Geometry check sheet. Reference: the model listing, model coordinates, mm. Give positions to 0.01 mm unless a question says otherwise; leave off trailing zeros. Order: outer loops, then holes, each group sorted by start corner. A loop starts at its lowest first (then second) coordinate and runs counter-clockwise, first axis right, second up. Notation, with made-up numbers: M 81,78.25 L 109,78.25 A22 ccw 109,93.25 Z; hole C 16.5,-32 d7. An arc over 180 degrees is marked long. Answer as a JSON object with one key per item and string values. Group by question number.
Autodesk Inventor part; units mm, degrees
ref_plane "YZ Plane" through (0, 0, 0) normal (1, 0, 0) x (0, 1, 0)
ref_plane "XZ Plane" through (0, 0, 0) normal (0, 1, 0) x (-1, 0, 0)
ref_plane "XY Plane" through (0, 0, 0) normal (0, 0, 1) x (1, 0, 0)
sketch "Sketch1" plane through (0, 0, 0) normal (0, 0, 1) x (1, 0, 0)
  line L0 (0, -7) -> (208, -7)
  line L1 (209, -8) -> (209, -30)
  line L2 (208, -31) -> (0, -31)
  line L3 (-1, -30) -> (-1, -8)
  circle A0 centre (38.25, -10.75) radius 1.75
  circle A1 centre (58.75, -10.75) radius 1.75
  circle A2 centre (149.25, -10.75) radius 1.75
  circle A3 centre (169.75, -10.75) radius 1.75
  circle A4 centre (38.25, -40.75) radius 1.75
  circle A5 centre (58.75, -40.75) radius 1.75
  circle A6 centre (149.25, -40.75) radius 1.75
  circle A7 centre (169.75, -40.75) radius 1.75
  arc A8 (0, -7) -> (-1, -8) centre (0, -8) ccw
  arc A9 (-1, -30) -> (0, -31) centre (0, -30) ccw
  arc A10 (208, -31) -> (209, -30) centre (208, -30) ccw
  arc A11 (209, -8) -> (208, -7) centre (208, -8) ccw
  point P0 (0, 0)
  point P1 (209, -31)
  point P2 (209, -7)
  point P3 (-1, -31)
  dimension "d0" = 210
  dimension "d1" = 24
  dimension "d10" = 111
  dimension "d13" = 30
  dimension "d16" = 1
extrude "Extrusion1" add sketch "Sketch1" along normal blind 2 contours L0 A11 L1 A10 L2 A9 L3 A8 | A0 | A1 | A2 | A3
sketch "Sketch2" plane through (0, 0, 2) normal (0, 0, 1) x (1, 0, 0)
  line L0 (209, -30) -> (209, -8)
  line L1 (209, -19) -> (-1, -19) construction
  line L2 (-1, -8) -> (-1, -30)
  line L3 (235.9536, -47.1551) -> (247.5417, -11.4905)
  line L4 (235.9536, -47.1551) -> (273.4536, -47.1551) construction
  line L5 (235.9536, -47.1551) -> (237.8557, -47.7731)
  line L6 (235.9536, -47.1551) -> (237.9536, -47.1551) construction
  line L7 (237.8557, -47.7731) -> (249.4438, -12.1085)
  line L8 (249.4438, -12.1085) -> (247.5417, -11.4905)
  line L9 (249.4438, -12.1085) -> (271.3181, -19.2159)
  line L10 (271.3181, -19.2159) -> (259.73, -54.8805)
  line L11 (259.73, -54.8805) -> (261.6321, -55.4986)
  line L12 (261.6321, -55.4986) -> (273.2202, -19.8339)
  line L13 (273.2202, -19.8339) -> (271.3181, -19.2159)
  line L14 (265.5241, -37.0482) -> (243.6498, -29.9408)
  line L15 (177.3204, -33.4945) -> (331.8534, -33.4945)
  line L16 (244.4446, -27.4945) -> (242.5425, -26.8765)
  line L17 (238.4427, -39.4945) -> (240.3448, -40.1125)
  line L18 (244.4446, -27.4945) -> (240.3448, -40.1125)
  line L19 (104, -19) -> (104, -19)
  line L20 (104, -19) -> (104, -19) construction
  line L21 (104, -20.25) -> (104, -17.75) construction
  line L22 (110.25, -20.25) -> (110.25, -17.75)
  line L23 (97.75, -17.75) -> (97.75, -20.25)
  arc A0 (97.75, -20.25) -> (110.25, -20.25) centre (104, -20.25) ccw
  arc A1 (110.25, -17.75) -> (97.75, -17.75) centre (104, -17.75) ccw
  line L24 (104, -19) -> (74, -19) construction
  line L25 (104, -19) -> (134, -19) construction
  line L26 (74, -20.25) -> (74, -17.75) construction
  line L27 (80.25, -20.25) -> (80.25, -17.75)
  line L28 (67.75, -17.75) -> (67.75, -20.25)
  arc A2 (67.75, -20.25) -> (80.25, -20.25) centre (74, -20.25) ccw
  arc A3 (80.25, -17.75) -> (67.75, -17.75) centre (74, -17.75) ccw
  line L29 (134, -20) -> (134, -18) construction
  line L30 (140.25, -20) -> (140.25, -18)
  line L31 (127.75, -18) -> (127.75, -20)
  arc A4 (127.75, -20) -> (140.25, -20) centre (134, -20) ccw
  arc A5 (140.25, -18) -> (127.75, -18) centre (134, -18) ccw
  line L32 (74, -19) -> (14, -19) construction
  line L33 (134, -19) -> (194, -19) construction
  line L34 (194, -20) -> (194, -18) construction
  line L35 (200.25, -20) -> (200.25, -18)
  line L36 (187.75, -18) -> (187.75, -20)
  arc A6 (187.75, -20) -> (200.25, -20) centre (194, -20) ccw
  arc A7 (200.25, -18) -> (187.75, -18) centre (194, -18) ccw
  line L37 (14, -20.25) -> (14, -17.75) construction
  line L38 (20.25, -20.25) -> (20.25, -17.75)
  line L39 (7.75, -17.75) -> (7.75, -20.25)
  arc A8 (7.75, -20.25) -> (20.25, -20.25) centre (14, -20.25) ccw
  arc A9 (20.25, -17.75) -> (7.75, -17.75) centre (14, -17.75) ccw
  circle A10 centre (14, -19) radius 10 construction
  line L40 (14, -19) -> (24.6066, -8.3934) construction
  line L41 (14, -19) -> (29, -19) construction
  line L42 (14, -19) -> (3.3934, -29.6066) construction
  circle A11 centre (4, -19) radius 1.75
  circle A12 centre (24, -19) radius 1.75
  circle A13 centre (54, -19) radius 1.75
  circle A14 centre (34, -19) radius 1.75
  circle A15 centre (84, -19) radius 1.75
  circle A16 centre (64, -19) radius 1.75
  circle A17 centre (114, -19) radius 1.75
  circle A18 centre (94, -19) radius 1.75
  circle A19 centre (144, -19) radius 1.75
  circle A20 centre (124, -19) radius 1.75
  circle A21 centre (174, -19) radius 1.75
  circle A22 centre (154, -19) radius 1.75
  circle A23 centre (204, -19) radius 1.75
  circle A24 centre (184, -19) radius 1.75
  point P0 (0, 0)
  point P1 (254.5869, -33.4945)
  dimension "d19" = 37.5
  dimension "d20" = 72
  dimension "d21" = 2
  dimension "d22" = 18
  dimension "d23" = 37.5
  dimension "d24" = 23
  dimension "d25" = 37.5
  dimension "d26" = 90
  dimension "d27" = 2
  dimension "d28" = 37.5
  dimension "d29" = 90
  dimension "d32" = 0
  dimension "d33" = 90
  dimension "d34" = 1.25
  dimension "d35" = 12.5
  dimension "d38" = 30
  dimension "d39" = 30
  dimension "d40" = 1.25
  dimension "d41" = 12.5
  dimension "d42" = 1
  dimension "d43" = 12.5
  dimension "d44" = 60
  dimension "d45" = 60
  dimension "d46" = 1
  dimension "d47" = 12.5
  dimension "d48" = 1.25
  dimension "d49" = 12.5
  dimension "d50" = 20
  dimension "d51" = 15
  dimension "d52" = 45
  dimension "d53" = 15
  dimension "d63" = 3.5
  dimension "d64" = 3.5
  dimension "d67" = 30
extrude "Extrusion2" cut sketch "Sketch2" against normal blind 10 contours A2 L28 A3 L27 | A4 L31 A5 L30 | A6 L36 A7 L35 | A8 L39 A9 L38 | A11 | A12 | A15 | A16 | A19 | A20 | A23 | A24
properties part number "Leg_Loadpipe_Plate" material "CFRP"
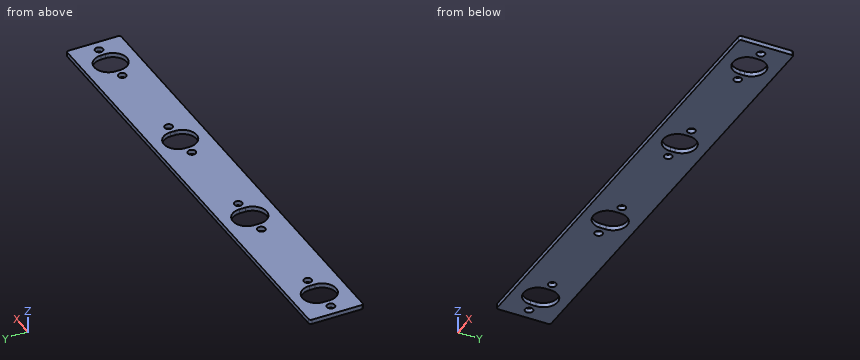
1. Thickness scan on line 1 along X through (y, z) = (-16, 1.9); line 2 along Y through (x, z) = (74, 0.1); line 3 along Y through (x, z) = (194, 0.4). Record the ranges inside material, lowest first. Write a range as [from, to].
2. Depth check by flat-ended pin: pin 1 (3 mm diameter, centred on x = 4, y = -19, fed in from +Z); pin 2 (8 mm diameter, centred on x = 44.5, y = -21.5, fed in from -Z). Enter the tip coordinate at first touch or a pass-through.
3. Cross-section at A-A (x = 64). Record the cut outline in (y, z).
4. Cross-section at C-C (x = 193.5). Record the cut outline in (y, z).
5. Cross-section at B-B (z = 1.25). State how many separate pieces and enclosed holes the cut face has, and give its area (3 significant figures).
Report:
{
 "1": {"line 1": "x = [-1, 8], [20, 68], [80, 128.08], [139.92, 188.08], [199.92, 209]", "line 2": "y = [-31, -26.5], [-11.5, -7]", "line 3": "y = [-31, -26.25], [-11.75, -7]"},
 "2": {"pin 1": "passes through", "pin 2": "stops at z = 0"},
 "3": {"outline": "M -31,0 L -20.75,0 L -20.75,2 L -31,2 Z; M -17.25,0 L -7,0 L -7,2 L -17.25,2 Z"},
 "4": {"outline": "M -31,0 L -26.23,0 L -26.23,2 L -31,2 Z; M -11.77,0 L -7,0 L -7,2 L -11.77,2 Z"},
 "5": {"separate pieces": "1", "enclosed holes": "12", "area": "4,360 mm2"}
}
